```python
from build123d import *

# Parameters (mm, degrees)
SKETCH1_W               = 76.2
SKETCH1_H               = 12.7
BOSS_EXTRUDE1_DEPTH     = 6.35
CUT_EXTRUDE1_DEPTH      = 1
CUT_EXTRUDE1_DEPTH_BACK = 7.35


with BuildPart() as part:
    # Sketch1 → Boss-Extrude1 (new body)
    with BuildSketch(Plane(origin=(0, 0, 0), x_dir=(1, 0, 0), z_dir=(0, 1, 0))):
        with Locations((38.1, -6.35)):
            Rectangle(SKETCH1_W, SKETCH1_H)
    extrude(amount=BOSS_EXTRUDE1_DEPTH)

    # Sketch2 → Cut-Extrude1 (cut, two sides)
    with BuildSketch(Plane(origin=(0, 0, 0), x_dir=(-1, 0, 0), z_dir=(0, -1, 0))) as cut_extrude1_sk:
        Polygon((-76.2, -8.6), (-76.2, -4.1), (-69.845872794, -4.1), (-69.845872794, -2.6), (-66.802, -2.6), (-66.802, -4.1), (-57.149530135, -4.1), (-57.149530135, -8.6), (-66.802, -8.6), (-66.802, -10.1), (-69.845872794, -10.1), (-69.845872794, -8.6), align=None)
        Polygon((-19.050469865, -4.1), (-9.398, -4.1), (-9.398, -2.6), (-6.354127206, -2.6), (-6.354127206, -4.1), (0, -4.1), (0, -8.6), (-6.354127206, -8.6), (-6.354127206, -10.1), (-9.398, -10.1), (-9.398, -8.6), (-19.050469865, -8.6), align=None)
    extrude(amount=CUT_EXTRUDE1_DEPTH, mode=Mode.SUBTRACT)
    extrude(cut_extrude1_sk.sketch, amount=-CUT_EXTRUDE1_DEPTH_BACK, mode=Mode.SUBTRACT)


solid = part.part
```
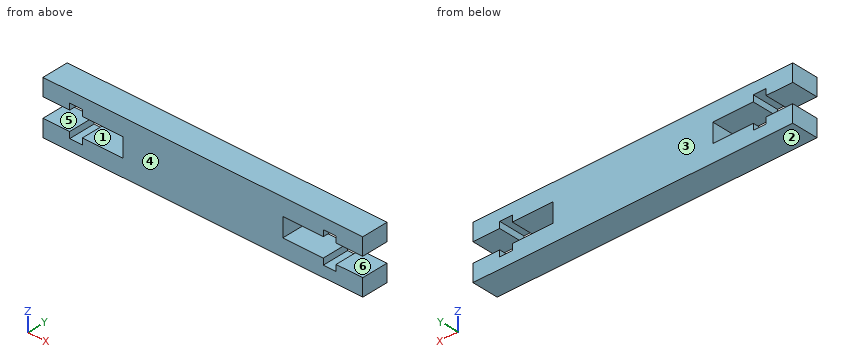
CAD build for the part. Positions are in the model's coordinates, mm. Face numbers are marked on the shaded views. A direction names the side the tool comes from. Coordinates: 2 decimals unless noted, no trailing zeros. Write each loop counter-clockwise with the first axis right and the second up, starting at its lowest first coordinate (ties: lowest second). Pieces come first, ordered by that corner, then holes.
(1) Cut at A-A, the plane x = 8. List the corners of the cut face in (y, z).
(2) Two-plate mould, pull along Z, no slides. Class the marked faces 1, 2 and 3: +Z half, -Z half, draft (parallel to the pull), parting line (faces both ways), or undercut.
(3) Flat gauge pins, fed straight in: pin 1 (1.6 mm diameter, centred on y = 4, z = 3, fed in from -X); pin 2 (3.5 mm diameter, centred on y = 3, z = 6, fed in from -X); pin 3 (2 mm diameter, centred on y = 3, z = 7, fed in from +X). Where does each tip first touch, or does it go through?
(4) Cut at B-B, the plane y = 4.5. List the corners of the cut face in (x, z), and give its area (3 significant figures).
(5) Cut at D-D, the plane z = 6.25. List the corners of the cut face in (x, y).
(6) 3-axis set-ups, long thin cutter, end or side, ignore diameter. For the marked faces 4, 5 and 6: which of +Z, -Z, +X, -X, +Y, -Y reach the whole face in a straight line?
(7) Drill centre lines: probe 1 along X at (y, z) = (2, 10); probe 2 along Z at (x, y) = (18, 3.25); probe 3 along X at (y, z) = (3, 7). Where is each one in solid material? Low to high.
(8) Cut at C-C, the plane x = 65. List the corners of the cut face in (y, z).
Geometry says:
1. outline: (0, 0) - (6.35, 0) - (6.35, 2.6) - (0, 2.6) - close; (0, 10.1) - (6.35, 10.1) - (6.35, 12.7) - (0, 12.7) - close
2. face 1: undercut
2. face 2: -Z half
2. face 3: draft
3. pin 1: stops at x = 0
3. pin 2: stops at x = 19.05
3. pin 3: stops at x = 57.15
4. outline: (0, 0) - (76.2, 0) - (76.2, 4.1) - (69.85, 4.1) - (69.85, 2.6) - (66.8, 2.6) - (66.8, 4.1) - (57.15, 4.1) - (57.15, 8.6) - (66.8, 8.6) - (66.8, 10.1) - (69.85, 10.1) - (69.85, 8.6) - (76.2, 8.6) - (76.2, 12.7) - (0, 12.7) - (0, 8.6) - (6.35, 8.6) - (6.35, 10.1) - (9.4, 10.1) - (9.4, 8.6) - (19.05, 8.6) - (19.05, 4.1) - (9.4, 4.1) - (9.4, 2.6) - (6.35, 2.6) - (6.35, 4.1) - (0, 4.1) - close
4. area: 778 mm2
5. outline: (19.05, 0) - (57.15, 0) - (57.15, 6.35) - (19.05, 6.35) - close
6. face 4: +Z, -Z, +X, -X, -Y
6. face 5: -X, +Y, -Y
6. face 6: +X, +Y, -Y
7. probe 1: x = 0 to 6.35, 9.4 to 66.8, 69.85 to 76.2
7. probe 2: z = 0 to 4.1, 8.6 to 12.7
7. probe 3: x = 19.05 to 57.15
8. outline: (0, 0) - (6.35, 0) - (6.35, 4.1) - (0, 4.1) - close; (0, 8.6) - (6.35, 8.6) - (6.35, 12.7) - (0, 12.7) - close
